For this review, take the finished solid that the model builds, in its own axes (mm). Face numbers are marked on the shaded views. Coordinates: 2 decimals unless noted, no trailing zeros. Order: outer loops, then holes, each group sorted by start corner. A loop starts at its lowest first (then second) coordinate and runs counter-clockwise, first axis right, second up. Notation, with made-up numbers: (47, 79.25) -> (72, 79.25) arc R11 ccw to (72, 87.25) -> close; hole circle Ø2 at (72.5, -7). An arc over 180 degrees is marked (long way). Write item = value, one per line. Start each with the question number.
1) Insertion check: pin 1 Ø1 at (y, z) = (0.5, 2) entering from -X; pin 2 Ø1 at (y, z) = (3.5, 0.5) entering from +X; pin 3 Ø4 at (x, y) = (-7.5, 16.5) entering from -Z. Each pin has a flat end and moves straight along its axis. Give the tip position at first contact, or say it passes through.
2) Consider section C-C on z = 3.25. Give the boundary of the cut face in (x, y).
3) Draft analysis for pull direction X (two halves, no side actions). For the marked faces 1, 2 and 3, state which applies: +X half, -X half, draft (parallel to the pull), parting line (faces both ways), or undercut.
4) Wall thickness on probe 1 along X at (y, z) = (-1, 2.7); probe 2 along Z at (x, y) = (-4, 2); probe 3 along X at (y, z) = (11.5, 3.15): over which ranges is each line inside the solid? List them lowest first. Write a range as [from, to].
from build123d import *

# Parameters (mm, degrees)
F1_DEPTH = 5
F2_SIZE  = 4.99999
F4_DEPTH = 2.5


# Not quite as in the source:
# - a fillet or chamfer is up to 0.001 mm smaller than in the source, because OpenCascade refuses the exact size


with BuildPart() as f1:
    # F0 (on Top) → F1 (new body)
    with BuildSketch(Plane.XY):
        Polygon((24.9973740429, 8.3822524399), (35, -11.5), (35, 47.5), (-35, 47.5), (-35, -14.74), (-20.0927332044, 15.4384202456), (-10.1515629949, -11.1895798258), (0, 0), (14.7012080997, -26.056649141), align=None)
        Polygon((35, 47.5), (35, -11.5), (40, -11.5), (40, 52.5), (-40, 52.5), (-40, -14.74), (-35, -14.74), (-35, 47.5), align=None)
    extrude(amount=F1_DEPTH)

    # F2 (size 5 in the source; OpenCascade refuses exactly that, so slightly less here)
    f2_edges = [f1.edges().sort_by_distance(p)[0] for p in [
        (40, 20.5, 0),
        (0, 52.5, 0),
        (-40, 18.88, 0),
    ]]
    chamfer(f2_edges, length=F2_SIZE)

    # F3 (on face) → F4 (cut)
    with BuildSketch(Plane(origin=(0, 0, 0), x_dir=(1, 0, 0), z_dir=(0, 0, -1))):
        with BuildLine():
            ThreePointArc((33.7950026252, 9.1048227638), (34.6974429309, 4.5921078013), (35, 0))
            Line((35, 0), (35, 11.5))
            Line((35, 11.5), (33.7950026252, 9.1048227638))
        make_face()
        with BuildLine():
            Line((-35, 14.74), (-35, 0))
            ThreePointArc((-35, 0), (-34.5462442763, 5.6175623185), (-33.1967424913, 11.0894674339))
            Line((-33.1967424913, 11.0894674339), (-35, 14.74))
        make_face()
        with BuildLine():
            ThreePointArc((-33.1967424913, 11.0894674339), (-34.5462442763, 5.6175623185), (-35, 0))
            ThreePointArc((-35, 0), (0, -35), (35, 0))
            ThreePointArc((35, 0), (34.6974429309, 4.5921078013), (33.7950026252, 9.1048227638))
            Line((33.7950026252, 9.1048227638), (24.9973740429, -8.3822524399))
            Line((24.9973740429, -8.3822524399), (14.7012080997, 26.056649141))
            Line((14.7012080997, 26.056649141), (0, 0))
            Line((0, 0), (-10.1515629949, 11.1895798258))
            Line((-10.1515629949, 11.1895798258), (-20.0927332044, -15.4384202456))
            Line((-20.0927332044, -15.4384202456), (-33.1967424913, 11.0894674339))
        make_face()
    extrude(amount=-F4_DEPTH, mode=Mode.SUBTRACT)


solid = f1.part
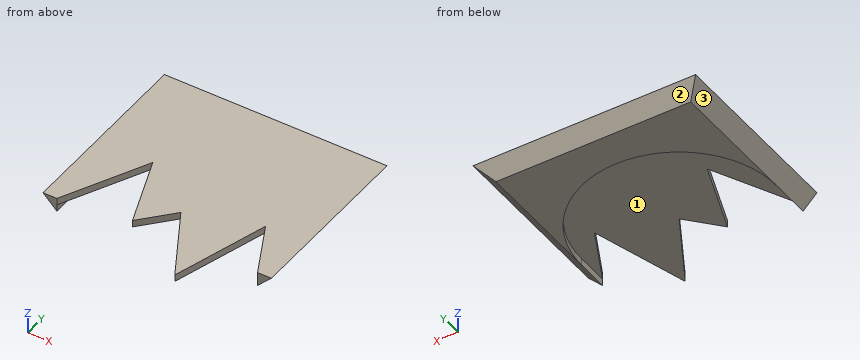
Answer sheet:
q1.pin_1 = -37.5
q1.pin_2 = 36
q1.pin_3 = 2.5
q2.outline = (-38.25, -14.74) -> (-35, -14.74) -> (-20.09, 15.44) -> (-10.15, -11.19) -> (0, 0) -> (14.7, -26.06) -> (25, 8.38) -> (35, -11.5) -> (38.25, -11.5) -> (38.25, 50.75) -> (-38.25, 50.75) -> close
q3.face_1 = undercut
q3.face_2 = draft
q3.face_3 = -X half
q4.probe_1 = [-37.7, -28.21], [-13.96, -0.91], [0.56, 22.19], [29.72, 37.7]
q4.probe_2 = [2.5, 5]
q4.probe_3 = [-38.15, -22.04], [-18.62, 38.15]
